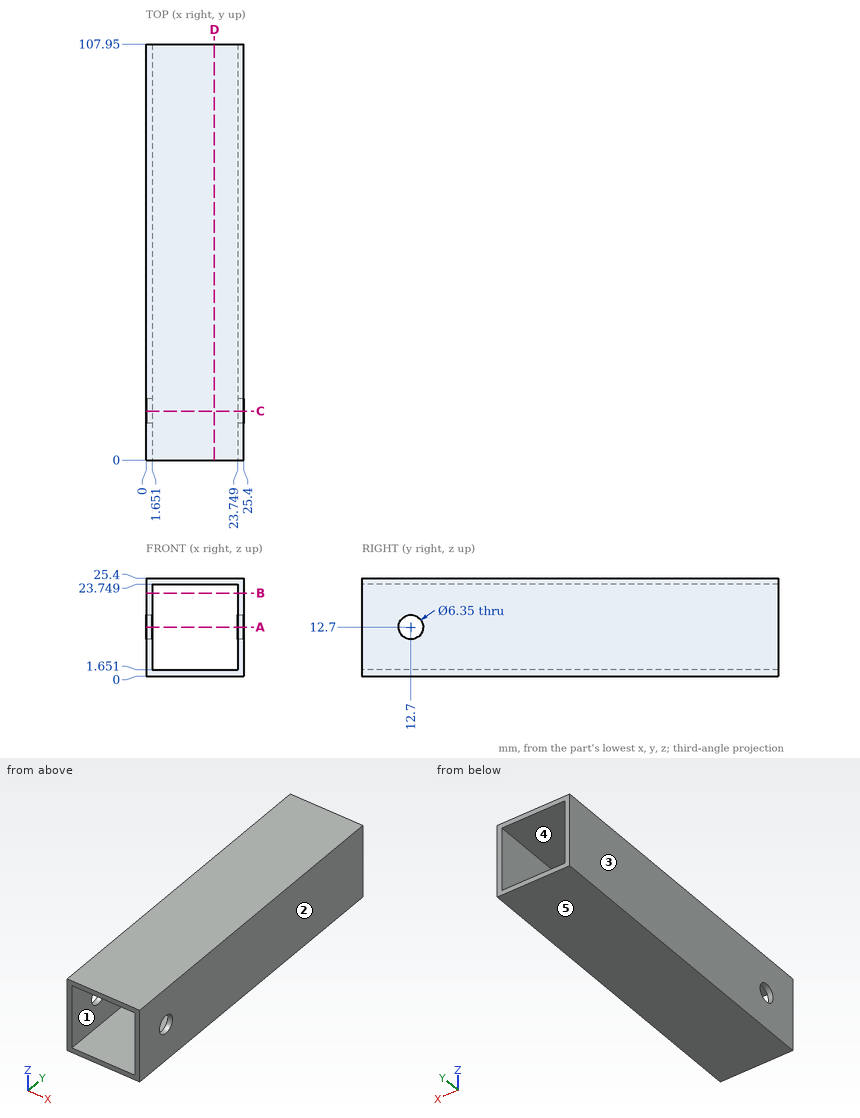
Can you work these out from the drawing? Everything is in mm from the part's minimum corner. A direction names the side the tool comes from. Give positions to 0.01 mm unless a question says otherwise; leave off trailing zeros. Order: outer loops, then holes, each group sorted by start corner. A loop starts at its lowest first (then second) coordinate and runs counter-clockwise, first axis right, second up.
1. I need wall thicknesses on L1, parallel to X at y = 79, z = 7.25; L2, parallel to Y at x = 24.4, z = 12.7 (3 decimals). Which ranges of each line are inside material? Lowest first, please.
2. Will these pins go through, and if not, where does the flat tip stop? P1, Ø7.5, axis at y = 12.7, z = 12.7, coming from the +X side; P2, Ø3, axis at x = 21, z = 8.5, coming from the +Y side.
3. Suppose I cut it at C-C (y = 12.7). List the corners of the cut face in (x, z) for me (3 decimals).
4. For the marked faces 4 and 5, which set-ups out of +Z, -Z, +X, -X, +Y, -Y let a thin tool reach every point of the face, with its end or its side?
5. Suppose I cut it at B-B (z = 21.5). List the corners of the cut face in (x, y) for me, plus the area to 3 significant figures.
6. Suppose I cut it at A-A (z = 12.7). List the corners of the cut face in (x, y) for me (3 decimals).
7. We'd pull the mould along X, two halves only. Please class the marked faces 1, 2 and 3: pulls with the +X half, pulls with the -X half, needs draft (parallel to the pull), parting line crosses it, or undercut.
8. Suppose I cut it at D-D (x = 17.75). List the corners of the cut face in (y, z) for me, plus the area to 3 significant figures.
Solved:
1. L1: x = 0 to 1.65, 23.75 to 25.4
1. L2: y = 0 to 9.525, 15.875 to 107.95
2. P1: stops at x = 25.4
2. P2: passes through
3. outline: (0, 0) - (25.4, 0) - (25.4, 9.525) - (23.749, 9.525) - (23.749, 1.651) - (1.651, 1.651) - (1.651, 9.525) - (0, 9.525) - close; (0, 15.875) - (1.651, 15.875) - (1.651, 23.749) - (23.749, 23.749) - (23.749, 15.875) - (25.4, 15.875) - (25.4, 25.4) - (0, 25.4) - close
4. face 4: +Y, -Y
4. face 5: -Z, +X, -X, +Y, -Y
5. outline: (0, 0) - (1.65, 0) - (1.65, 107.95) - (0, 107.95) - close; (23.75, 0) - (25.4, 0) - (25.4, 107.95) - (23.75, 107.95) - close
5. area: 356 mm2
6. outline: (0, 0) - (1.651, 0) - (1.651, 9.525) - (0, 9.525) - close; (0, 15.875) - (1.651, 15.875) - (1.651, 107.95) - (0, 107.95) - close; (23.749, 0) - (25.4, 0) - (25.4, 9.525) - (23.749, 9.525) - close; (23.749, 15.875) - (25.4, 15.875) - (25.4, 107.95) - (23.749, 107.95) - close
7. face 1: undercut
7. face 2: pulls with the +X half
7. face 3: pulls with the -X half
8. outline: (0, 0) - (107.95, 0) - (107.95, 1.65) - (0, 1.65) - close; (0, 23.75) - (107.95, 23.75) - (107.95, 25.4) - (0, 25.4) - close
8. area: 356 mm2
